```python
from build123d import *

# Parameters (mm, degrees)
SKETCH_1_W          = 10
SKETCH_1_H          = 10
SKETCH_1_W_2        = 6.4
SKETCH_1_H_2        = 6.4
EXTRUDE_1_DEPTH     = 160
SKETCH_2_R          = 1.5
CUT_EXTRUDE_1_DEPTH = 161.390149323
SKETCH_3_R          = 1.5
CUT_EXTRUDE_2_DEPTH = 161.390149323
SKETCH_4_R          = 1.5
CUT_EXTRUDE_3_DEPTH = 161.390149323


with BuildPart() as part:
    # 草图1 → 凸台-拉伸1 (new, symmetric)
    with BuildSketch(Plane(origin=(0, 0, 0), x_dir=(1, 0, 0), z_dir=(0, 1, 0))):
        Rectangle(SKETCH_1_W, SKETCH_1_H)
        Rectangle(SKETCH_1_W_2, SKETCH_1_H_2, mode=Mode.SUBTRACT)
    extrude(amount=EXTRUDE_1_DEPTH, both=True)

    # 草图2 → 切除-拉伸1 (cut, through all)
    with BuildSketch(Plane(origin=(0, 0, -5), x_dir=(-1, 0, 0), z_dir=(0, 0, -1))):
        with Locations((0, -149.7)):
            Circle(SKETCH_2_R)
        with Locations((0, -139.7)):
            Circle(SKETCH_2_R)
        with Locations((0, -129.7)):
            Circle(SKETCH_2_R)
        with Locations((0, 139.7)):
            Circle(SKETCH_2_R)
        with Locations((0, 149.7)):
            Circle(SKETCH_2_R)
        with Locations((0, 129.7)):
            Circle(SKETCH_2_R)
    extrude(amount=-CUT_EXTRUDE_1_DEPTH, mode=Mode.SUBTRACT)

    # 草图3 → 切除-拉伸2 (cut, through all)
    with BuildSketch(Plane.ZY.offset(5)):
        with Locations((0, -110.7)):
            Circle(SKETCH_3_R)
        with Locations((0, -100.7)):
            Circle(SKETCH_3_R)
        with Locations(Location((0, 100.7, 0), (0, 0, 180))):
            Circle(SKETCH_3_R)
        with Locations(Location((0, 110.7, 0), (0, 0, 180))):
            Circle(SKETCH_3_R)
    extrude(amount=-CUT_EXTRUDE_2_DEPTH, mode=Mode.SUBTRACT)

    # 草图4 → 切除-拉伸3 (cut, through all)
    with BuildSketch(Plane(origin=(5, 0, 0), x_dir=(0, 0, -1), z_dir=(1, 0, 0))):
        Circle(SKETCH_4_R)
        with Locations((0, -10)):
            Circle(SKETCH_4_R)
        with Locations((0, 10)):
            Circle(SKETCH_4_R)
    extrude(amount=-CUT_EXTRUDE_3_DEPTH, mode=Mode.SUBTRACT)


solid = part.part
```
Model file for the job. Use its own axes, mm. A direction names the side the tool comes from. Coordinates: 2 decimals unless noted, no trailing zeros. Write each loop counter-clockwise with the first axis right and the second up, starting at its lowest first coordinate (ties: lowest second). Pieces come first, ordered by that corner, then holes. Notation, with made-up numbers: (69, -37) - (76, -37) arc R14 ccw to (76, -31) - close; hole circle Ø10 at (2, 68). An arc over 180 degrees is marked (long way). One line per item, written item: value. Start each with the question number.
1. Mould opens along X. For faces 1 (the flat face through (0, 2, -3.2)), 2 (the flat face through (-5, 2, 0)), 3 (the flat face through (0, 2, -5)) say: released by +X, released by -X, zero draft, split by the parting line, or undercut.
2. Probe line 1 (X direction, y = 80, z = 3); line 2 (Z direction, x = 3.75, y = -100.7). List the from-to ranges inside material, lowest first. Write a range as from..to.
3. Flat gauge pins, fed straight in: pin 1 (2.5 mm diameter, centred on y = -110.7, z = 0, fed in from +X); pin 2 (5 mm diameter, centred on y = -110.7, z = 0, fed in from +X). Where does each tip first touch, or does it go through?
4. Slice it at A-A (y = 77). Write the cut outline in (x, z).
5. Tool access for faces 4 (the flat face through (-3.2, 2, 0)), 5 (the flat face through (-0.1, 160, -3.4)): list every direction of +Z, -Z, +X, -X, +Y, -Y with a clear straight run to the whole face (end or side of a thin tool).
6. Slice it at B-B (z = 0). Count the separate pieces of the cut face and the enclosed holes in it, plus the area to 3 significant figures.
Answers below:
1. face 1: undercut
1. face 2: released by -X
1. face 3: zero draft
2. line 1: x = -5..-3.2, 3.2..5
2. line 2: z = -5..-1.5, 1.5..5
3. pin 1: passes through
3. pin 2: stops at x = 5
4. outline: (-5, -5) - (5, -5) - (5, 5) - (-5, 5) - close; hole (-3.2, -3.2) - (3.2, -3.2) - (3.2, 3.2) - (-3.2, 3.2) - close
5. face 4: +Y, -Y
5. face 5: +Z, -Z, +X, -X, +Y
6. separate pieces: 16
6. enclosed holes: 0
6. area: 1,080 mm^2
